Geometry check sheet. Reference: the model listing, model coordinates, mm. Face numbers are marked on the shaded views. Coordinates: 2 decimals unless noted, no trailing zeros. Write each loop counter-clockwise with the first axis right and the second up, starting at its lowest first coordinate (ties: lowest second). Pieces come first, ordered by that corner, then holes. Notation, with made-up numbers: M 77.5,-32.75 L 135.5,-32.75 A16 cw 135.5,-27.75 Z; hole C 17,41 d11. An arc over 180 degrees is marked long. Write each question's results on one line, items separated by ' | '.
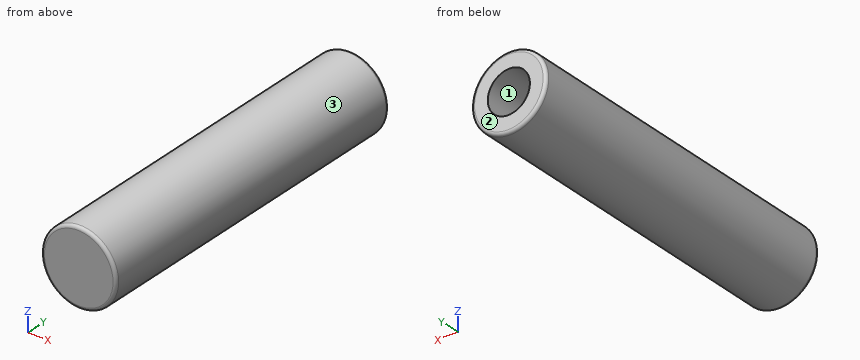
```python
from build123d import *

# Parameters (mm, degrees)
F_1_2_13_TAPPED_HOLE1_D     = 10.71626
F_1_2_13_TAPPED_HOLE1_DEPTH = 19.05
F_1_2_13_TAPPED_HOLE1_TIP   = 3.219489309


with BuildPart() as part:
    # Sketch1 → Revolve1 (revolve)
    with BuildSketch(Plane.XY):
        with BuildLine():
            Line((0, 0), (0, 87.3506))
            Line((0, 87.3506), (8.73125, 87.3506))
            ThreePointArc((8.73125, 87.3506), (9.292516008, 87.118116008), (9.525, 86.55685))
            Line((9.525, 86.55685), (9.525, 0.79375))
            ThreePointArc((9.525, 0.79375), (9.292516008, 0.232483992), (8.73125, 0))
            Line((8.73125, 0), (0, 0))
        make_face()
    revolve(axis=Axis((0, 288.392157732, 0), (0, -1, 0)))

    # 1/2-13 Tapped Hole1
    with Locations(Plane(origin=(0, 87.3506, 0), x_dir=(1, 0, 0), z_dir=(0, 1, 0))):
        with Locations((0, 0)):
            Hole(F_1_2_13_TAPPED_HOLE1_D / 2, depth=F_1_2_13_TAPPED_HOLE1_DEPTH)
            with Locations((0, 0, -(F_1_2_13_TAPPED_HOLE1_DEPTH + F_1_2_13_TAPPED_HOLE1_TIP / 2))):  # 118° drill point
                Cone(0, F_1_2_13_TAPPED_HOLE1_D / 2, F_1_2_13_TAPPED_HOLE1_TIP, mode=Mode.SUBTRACT)


solid = part.part
```
Q1. Sectioned sample at C-C on y = 67.5. Record the cut outline in (x, z) (3 decimals), and give its area (3 significant figures).
Geometry check:
outline: C 0,0 d19.05; hole C 0,0 d8.051 | area: 234 mm2
Q2. Mould release check, pull along Z, two halves, no side actions. Record for the marked faces 1, 2 and 3: pulls with the +Z half, pulls with the -Z half, needs draft (parallel to the pull), parting line crosses it, or undercut.
Geometry check:
face 1: undercut | face 2: needs draft | face 3: parting line crosses it
Q3. Depth check by flat-ended pin: P1, Ø5, axis at y = 15.5, z = 4, coming from the -X side; P2, Ø2, axis at x = -2, z = 2.5, coming from the +Y side; P3, Ø1, axis at x = 0, z = 1.5, coming from the +Y side. Enter the tip coordinate at first touch or a pass-through.
Geometry check:
P1: stops at x = -9.41 | P2: stops at y = 67.61 | P3: stops at y = 66.28
Q4. Scan lines: probe 1 along Z at (x, y) = (0, 77.25) (3 decimals); probe 2 along X at (y, z) = (70.5, -1); probe 3 along X at (y, z) = (32, -0.5). Record each from-to range of solid material in increasing order.
Geometry check:
probe 1: z = -9.525 to -5.358, 5.358 to 9.525 | probe 2: x = -9.47 to -5.26, 5.26 to 9.47 | probe 3: x = -9.51 to 9.51
Q5. Sectioned sample at B-B on y = 35. Record the cut outline in (x, z) (3 decimals), and give its area (3 significant figures).
Geometry check:
outline: C 0,0 d19.05 | area: 285 mm2
Q6. Sectioned sample at A-A on y = 78. Record the cut outline in (x, z) (3 decimals), and give its area (3 significant figures).
Geometry check:
outline: C 0,0 d19.05; hole C 0,0 d10.716 | area: 195 mm2
